Read the model definition and answer for the solid it produces. Units are mm, in the model's axes. A direction names the side the tool comes from. Coordinates: 2 decimals unless noted, no trailing zeros. Write each loop counter-clockwise with the first axis right and the second up, starting at its lowest first coordinate (ties: lowest second). Pieces come first, ordered by that corner, then holes. Notation, with made-up numbers: (-9.75, -2.75) -> (43.25, -2.75) arc R26 ccw to (43.25, 32.25) -> close; hole circle Ø5 at (23, 19.5). An arc over 180 degrees is marked (long way). Answer in a Markdown table with one row per item. Add a question column.
Item 1: Given pin 1 Ø10 at (x, y) = (-5, 1.5) entering from -Z, flat-ended and moving along its own axis, determine where the tip first touches the part or whether it passes through.
Item 2: Which of the six approach directions +Z, -Z, +X, -X, +Y, -Y give full straight-line access (tool end or side, diameter ignored) to faces 1 (the face through (-12.5, 0, 394)), 2 (the face through (-9.5, 0, 394))?
Item 3: Section A-A on y = -1.25 is taken. Write down the section's boundary in (x, z).
Item 4: Section B-B on x = -0.75 is taken. Write down the section's boundary in (y, z).
Item 5: For a pull along X with two mould halves and no side action, classify faces 3 (the face through (0, 9.5, 395)), 4 (the face through (12.5, 0, 394)), 5 (the face through (-11, 0, 800)) as +X half, -X half, draft (parallel to the pull), parting line (faces both ways), or undercut.
Item 6: Straight lines are drawn through the part: line 1 (Y direction, x = -6.5, z = 448.5); line 2 (X direction, y = 7, z = 70); line 3 (X direction, y = 9, z = 586). For each, find the intervals that lie inside material, in ascending order. Write a range as from..to.
Item 7: Section C-C on z = 125.5 is taken. Write down the section's boundary in (x, y).
Autodesk Inventor part; units mm, degrees
ref_plane "Start plane" through (0, 0, -12.5) normal (0, 0, 1) x (1, 0, 0)
ref_plane "End plane" through (0, 0, 812.5) normal (0, 0, 1) x (1, 0, 0)
ref_plane "Work Plane4" through (0, -12.5, 812.5) normal (0, 0.7071, 0.7071) x (1, 0, 0)
ref_plane "Start plane" through (0, 0, -12.5) normal (0, 0, 1) x (1, 0, 0)
ref_plane "End plane" through (0, 0, 812.5) normal (0, 0, 1) x (1, 0, 0)
sketch "Sketch" plane through (0, 0, 0) normal (0, 0, 1) x (1, 0, 0)
  line L0 (-12.5, -6.5) -> (-12.5, 6.5)
  line L1 (-6.5, 12.5) -> (6.5, 12.5)
  line L2 (12.5, 6.5) -> (12.5, -6.5)
  line L3 (6.5, -12.5) -> (-6.5, -12.5)
  arc A0 (-12.5, -6.5) -> (-6.5, -12.5) centre (-6.5, -6.5) ccw
  arc A1 (-6.5, 12.5) -> (-12.5, 6.5) centre (-6.5, 6.5) ccw
  arc A2 (12.5, 6.5) -> (6.5, 12.5) centre (6.5, 6.5) ccw
  arc A3 (6.5, -12.5) -> (12.5, -6.5) centre (6.5, -6.5) ccw
  arc A4 (-6.5, 9.5) -> (-9.5, 6.5) centre (-6.5, 6.5) ccw
  line L4 (-6.5, 9.5) -> (6.5, 9.5)
  arc A5 (9.5, 6.5) -> (6.5, 9.5) centre (6.5, 6.5) ccw
  line L5 (9.5, 6.5) -> (9.5, -6.5)
  arc A6 (6.5, -9.5) -> (9.5, -6.5) centre (6.5, -6.5) ccw
  line L6 (6.5, -9.5) -> (-6.5, -9.5)
  arc A7 (-9.5, -6.5) -> (-6.5, -9.5) centre (-6.5, -6.5) ccw
  line L7 (-9.5, -6.5) -> (-9.5, 6.5)
  line L8 (0, 19.2397) -> (0, -19.2397) construction
  line L9 (-19.2397, 0) -> (19.2397, 0) construction
  dimension "d7" = 6
  dimension "d10" = 25
  dimension "d11" = 25
  dimension "d12" = 3
  dimension "d15" = 12.5
  dimension "d16" = 12.5
extrude "Body" add sketch "Sketch" along normal up to surface (825 mm away) from surface at -12.5
sketch "Sketch3" plane through (0, 0, 0) normal (0, 0, 1) x (1, 0, 0)
  line L0 (0, 0) -> (10, 0)
ref_plane "Work Plane3" through (0, 0, 0) normal (0, -1, 0) x (1, 0, 0)
sketch "Sketch4" plane through (0, 0, 0) normal (0, -1, 0) x (1, 0, 0)
  line L0 (-2, -12.5) -> (12, -12.5)
  line L1 (-2, 812.5) -> (12, 812.5)
  dimension "d18" = 825
ref_plane "Work Plane4" through (0, -12.5, 812.5) normal (0, 0.7071, 0.7071) x (1, 0, 0)
split "Split1" plane through (0, -12.5, 812.5) removes the side toward (0, 0.7071, 0.7071)
ref_plane "Work Plane5" through (0, -12.5, -12.5) normal (0, 0.7071, -0.7071) x (1, 0, 0)
split "Split2" plane through (0, -12.5, -12.5) removes the side toward (0, 0.7071, -0.7071)
equation "\"d7\" = G_IR"
equation "\"d10\" = G_H"
equation "\"d11\" = G_W"
equation "\"d12\" = G_T"
equation "\"d15\" = 0.5 * d10"
equation "\"d16\" = 0.5 * d11"
equation "\"d3\" = G_L"
equation "\"G_W\" = 25"
equation "\"G_H\" = 25"
equation "\"G_T\" = 3"
equation "\"G_IR\" = 6"
equation "\"G_L\" = d18"
equation "\"G_OFFSET_START\" = 12.5"
equation "\"G_OFFSET_END\" = 12.5"
equation "\"d13\" = -G_OFFSET_START"
equation "\"d14\" = G_OFFSET_END + B_L"
properties part number "AS 1163 - C350L0 25x25x3.0 SHS - 825" material "Steel, Mild"
Results below:
| question | item | result |
|---|---|---|
| 1 | pin 1 | stops at z = -0.68 |
| 2 | face 1 | +Z, -Z, -X, +Y, -Y |
| 2 | face 2 | +Z, -Z |
| 3 | outline | (-12.5, -1.25) -> (-9.5, -1.25) -> (-9.5, 801.25) -> (-12.5, 801.25) -> close; (9.5, -1.25) -> (12.5, -1.25) -> (12.5, 801.25) -> (9.5, 801.25) -> close |
| 4 | outline | (-12.5, -12.5) -> (-9.5, -9.5) -> (-9.5, 809.5) -> (-12.5, 812.5) -> close; (9.5, 9.5) -> (12.5, 12.5) -> (12.5, 787.5) -> (9.5, 790.5) -> close |
| 5 | face 3 | undercut |
| 5 | face 4 | +X half |
| 5 | face 5 | draft |
| 6 | line 1 | y = -12.5..-9.5, 9.5..12.5 |
| 6 | line 2 | x = -12.48..-9.46, 9.46..12.48 |
| 6 | line 3 | x = -11.95..-8.16, 8.16..11.95 |
| 7 | outline | (-12.5, -6.5) arc R6 ccw to (-6.5, -12.5) -> (6.5, -12.5) arc R6 ccw to (12.5, -6.5) -> (12.5, 6.5) arc R6 ccw to (6.5, 12.5) -> (-6.5, 12.5) arc R6 ccw to (-12.5, 6.5) -> close; hole (-9.5, -6.5) arc R3 ccw to (-6.5, -9.5) -> (6.5, -9.5) arc R3 ccw to (9.5, -6.5) -> (9.5, 6.5) arc R3 ccw to (6.5, 9.5) -> (-6.5, 9.5) arc R3 ccw to (-9.5, 6.5) -> close |
